from build123d import *

# Parameters (mm, degrees)
BASE_FLANGE1_DEPTH = 20
CUT_EXTRUDE1_REACH = 48.393
SKETCH6_R          = 1.5
FILLET1_R          = 3
FILLET2_R          = 3
CUT_EXTRUDE4_DEPTH = 85.132737956


# Sheet-metal steps are written as plain solids
with BuildPart() as part:
    # Sketch1 → Base-Flange1 (new body)
    with BuildSketch(Plane(origin=(0, 0, 0), x_dir=(1, 0, 0), z_dir=(0, 1, 0))):
        with BuildLine():
            Line((-9.340010949, 80.332543816), (-9.340010949, 41.069143816))
            ThreePointArc((-9.340010949, 41.069143816), (-9.124265804, 40.548288961), (-8.603410949, 40.332543816))
            Line((-8.603410949, 40.332543816), (5.659989051, 40.332543816))
            Line((5.659989051, 40.332543816), (5.659989051, 37.332543816))
            Line((5.659989051, 37.332543816), (-8.603410949, 37.332543816))
            ThreePointArc((-8.603410949, 37.332543816), (-11.245586147, 38.426968618), (-12.340010949, 41.069143816))
            Line((-12.340010949, 41.069143816), (-12.340010949, 80.332543816))
            Line((-12.340010949, 80.332543816), (-9.340010949, 80.332543816))
        make_face()
    extrude(amount=BASE_FLANGE1_DEPTH)

    # Sketch6 → Cut-Extrude1 (cut, up to next)
    with BuildSketch(Plane(origin=(0, 0, -40.332543816), x_dir=(-1, 0, 0), z_dir=(0, 0, -1)), mode=Mode.PRIVATE) as cut_extrude1_sk1:
        with Locations((-0.659989051, 16)):
            Circle(SKETCH6_R)
    cut_extrude1_tool1 = extrude(cut_extrude1_sk1.sketch, amount=-CUT_EXTRUDE1_REACH, mode=Mode.PRIVATE) & part.part
    # Sketch6 → Cut-Extrude1 (cut, up to next)
    with BuildSketch(Plane(origin=(0, 0, -40.332543816), x_dir=(-1, 0, 0), z_dir=(0, 0, -1)), mode=Mode.PRIVATE) as cut_extrude1_sk2:
        with Locations((-0.659989051, 4)):
            Circle(SKETCH6_R)
    cut_extrude1_tool2 = extrude(cut_extrude1_sk2.sketch, amount=-CUT_EXTRUDE1_REACH, mode=Mode.PRIVATE) & part.part
    add(cut_extrude1_tool1.solids().sort_by_distance((0.659989, 16, -40.332544))[0], mode=Mode.SUBTRACT)
    add(cut_extrude1_tool2.solids().sort_by_distance((0.659989, 4, -40.332544))[0], mode=Mode.SUBTRACT)

    # Fillet1
    fillet1_edges = [part.edges().sort_by_distance(p)[0] for p in [
        (5.659989051, 20, -38.832543816),
        (5.659989051, 0, -38.832543816),
    ]]
    fillet(fillet1_edges, radius=FILLET1_R)

    # Fillet2
    fillet2_edges = [part.edges().sort_by_distance(p)[0] for p in [
        (-10.840010949, 20, -80.332543816),
        (-10.840010949, 0, -80.332543816),
    ]]
    fillet(fillet2_edges, radius=FILLET2_R)

    # Sketch7 → Cut-Extrude4 (cut, through all)
    with BuildSketch(Plane(origin=(-9.340010949, 0, 0), x_dir=(0, 0, -1), z_dir=(1, 0, 0))):
        with BuildLine():
            Line((72.569143816, 11.1), (72.569143816, 9.7))
            ThreePointArc((72.569143816, 9.7), (71.069143816, 8.2), (69.569143816, 9.7))
            Line((69.569143816, 9.7), (69.569143816, 11.1))
            ThreePointArc((69.569143816, 11.1), (71.069143816, 12.6), (72.569143816, 11.1))
        make_face()
        with BuildLine():
            Line((72.569143816, 4.4), (72.569143816, 3))
            ThreePointArc((72.569143816, 3), (71.069143816, 1.5), (69.569143816, 3))
            Line((69.569143816, 3), (69.569143816, 4.4))
            ThreePointArc((69.569143816, 4.4), (71.069143816, 5.9), (72.569143816, 4.4))
        make_face()
    extrude(amount=-CUT_EXTRUDE4_DEPTH, mode=Mode.SUBTRACT)


solid = part.part
Could you check a few things on this model? Use its own coordinates, in mm. A direction names the side the tool comes from. Coordinates: 2 decimals unless noted, no trailing zeros. Write each loop counter-clockwise with the first axis right and the second up, starting at its lowest first coordinate (ties: lowest second). Pieces come first, ordered by that corner, then holes. Notation, with made-up numbers: (49.5, 78) - (98.5, 78) arc R20 ccw to (98.5, 102) - close; hole circle Ø4 at (28, 63.5). An arc over 180 degrees is marked (long way). Write item = value, one per line.
1) Suppose I cut it at A-A on y = 16. Please give me the cut outline in (x, z).
Result set:
outline = (-12.34, -80.33) - (-9.34, -80.33) - (-9.34, -41.07) arc R0.74 cw to (-8.6, -40.33) - (-0.84, -40.33) - (-0.84, -37.33) - (-8.6, -37.33) arc R3.74 ccw to (-12.34, -41.07) - close; (2.16, -40.33) - (5.66, -40.33) - (5.66, -37.33) - (2.16, -37.33) - close
2) We'd pull the mould along X, two halves only. Please class faces 4 (the cylindrical face through (-0.146, 5.265, -38.854)), 5 (the flat face through (-1, 10, -37.333)), 6 (the flat face through (-12.34, 10, -60)): +X half, -X half, draft (parallel to the pull), parting line (faces both ways), or undercut.
Result set:
face_4 = undercut
face_5 = draft
face_6 = -X half
3) Suppose I cut it at C-C on y = 13.25. Please give me the cut outline in (x, z), plus the area to 3 significant figures.
Result set:
outline = (-12.34, -80.33) - (-9.34, -80.33) - (-9.34, -41.07) arc R0.74 cw to (-8.6, -40.33) - (5.66, -40.33) - (5.66, -37.33) - (-8.6, -37.33) arc R3.74 ccw to (-12.34, -41.07) - close
area = 171 mm2
4) Will these pins go through, and if not, where does the flat tip stop? pin 1 Ø3.5 at (x, y) = (0.66, 16) entering from +Z; pin 2 Ø7 at (x, y) = (-5, 7) entering from -Z; pin 3 Ø1.5 at (y, z) = (11, -71.5) entering from -X; pin 4 Ø6 at (y, z) = (3, -64) entering from +X.
Result set:
pin_1 = -37.33
pin_2 = -40.33
pin_3 = through
pin_4 = -9.34
5) Suppose I cut it at B-B on z = -65. Please give me the cut outline in (x, y), plus the area to 3 significant figures.
Result set:
outline = (-12.34, 0) - (-9.34, 0) - (-9.34, 20) - (-12.34, 20) - close
area = 60.0 mm2
6) Please list where these lines run through material, in increasing order: line 1 (X direction, y = 13.5, z = -61.5); line 2 (Z direction, x = -6.25, y = 4.75); line 3 (Z direction, x = -10.75, y = 2). Write a range as [from, to].
Result set:
line_1 = [-12.34, -9.34]
line_2 = [-40.33, -37.33]
line_3 = [-80.16, -72.19], [-69.95, -38.01]
7) For faces 1 (the cylindrical face through (-10.8, 8.2, -71.1)), 2 (the cylindrical face through (-10.819, 19.098, -79.477)), 3 (the flat face through (-2, 10, -40.333)), which set-ups out of +Z, -Z, +X, -X, +Y, -Y let a thin tool reach every point of the face, with its end or its side?
Result set:
face_1 = +X, -X
face_2 = -Z, +X, -X, +Y
face_3 = -Z, +X, +Y, -Y
8) Suppose I cut it at D-D on x = -5.5. Please give me the cut outline in (y, z).
Result set:
outline = (0, -40.33) - (20, -40.33) - (20, -37.33) - (0, -37.33) - close
